Check sheet for the modelled part. Datum: model origin and axes. Units: mm. A direction names the side the tool comes from. Give positions to 0.01 mm unless a question says otherwise; leave off trailing zeros. Loops run counter-clockwise (first coordinate to the right, second up) from the corner with the lowest first, then second, coordinate; pieces in that order, holes last. Notation, with made-up numbers: M 46,-14.75 L 54,-14.75 A24 cw 54,15.25 Z; hole C 46.25,80.25 d3. An arc over 180 degrees is marked long. One line per question, with ' | ' between items. Start each with the question number.
from build123d import *

# Parameters (mm, degrees)
CUT_EXTRUDE1_START     = -4
CUT_EXTRUDE1_OUTLINE_R = 1
CUT_EXTRUDE1_DEPTH     = 4
SKETCH3_R              = 1
CUT_EXTRUDE2_DEPTH     = 3


# Read off the part's stored shape, not the designer's step: Cut-Extrude1
with BuildPart() as part:
    # Sketch1 → Revolve1 (revolve)
    with BuildSketch(Plane.XY, mode=Mode.PRIVATE) as revolve1_sk:
        Polygon((0, 22), (0, -1.8), (1, -1.8), (1, 0), (9.5, 0), (11.5, 2), (11.5, 3), (11, 3), (11, 3.5), (11.5, 3.5), (11.5, 4.5), (9.5, 4.5), (9.5, 4.8), (11.5, 4.8), (11.5, 14.5), (7.5, 18.5), (1, 18.5), (1, 22), align=None)
        Polygon((2, 17.5), (7.085786438, 17.5), (10.5, 14.085786438), (10.5, 11.635505843), (1, 11.635505843), (1, 16.5), (2, 16.5), align=None, mode=Mode.SUBTRACT)
    revolve(revolve1_sk.sketch.rotate(Axis((0, 22, 0), (0, -1, 0)), 180), axis=Axis((0, 22, 0), (0, -1, 0)))

    # Cut-Extrude1 outline → Cut-Extrude1 (cut)
    with BuildSketch(Plane(origin=(0, 18.5, 0), x_dir=(1, 0, 0), z_dir=(0, 1, 0)).offset(CUT_EXTRUDE1_START)):
        with BuildLine():
            Line((-3, 14.723214578), (-3, 9))
            ThreePointArc((-3, 9), (-2.83069097, 8.006426333), (-2.341874246, 7.124999996))
            ThreePointArc((-2.341874246, 7.124999996), (0, 7.5), (2.341874249, 7.125))
            ThreePointArc((2.341874249, 7.125), (2.830690966, 8.006426323), (3, 9))
            Line((3, 9), (3, 14.723214578))
            Line((3, 14.723214578), (-3, 14.723214578))
        make_face()
        with BuildLine():
            Line((11.25067785, 9.9596835), (6.294228634, 7.098076211))
            ThreePointArc((6.294228634, 7.098076211), (5.518423113, 6.454663457), (4.999493876, 5.590622588))
            ThreePointArc((4.999493876, 5.590622588), (6.495190528, 3.75), (7.341368127, 1.534377408))
            ThreePointArc((7.341368127, 1.534377408), (8.349114075, 1.551762875), (9.294228634, 1.901923789))
            Line((9.294228634, 1.901923789), (14.25067785, 4.763531077))
            Line((14.25067785, 4.763531077), (11.25067785, 9.9596835))
        make_face()
        with BuildLine():
            Line((14.25067785, -4.763531077), (9.294228634, -1.901923789))
            ThreePointArc((9.294228634, -1.901923789), (8.349114084, -1.551762876), (7.341368122, -1.534377408))
            ThreePointArc((7.341368122, -1.534377408), (6.495190528, -3.75), (4.999493877, -5.590622592))
            ThreePointArc((4.999493877, -5.590622592), (5.518423107, -6.45466345), (6.294228634, -7.098076211))
            Line((6.294228634, -7.098076211), (11.25067785, -9.9596835))
            Line((11.25067785, -9.9596835), (14.25067785, -4.763531077))
        make_face()
        with BuildLine():
            Line((3, -14.723214578), (3, -9))
            ThreePointArc((3, -9), (2.83069097, -8.006426333), (2.341874246, -7.124999996))
            ThreePointArc((2.341874246, -7.124999996), (0, -7.5), (-2.341874249, -7.125))
            ThreePointArc((-2.341874249, -7.125), (-2.830690966, -8.006426323), (-3, -9))
            Line((-3, -9), (-3, -14.723214578))
            Line((-3, -14.723214578), (3, -14.723214578))
        make_face()
        with BuildLine():
            Line((-11.25067785, -9.9596835), (-6.294228634, -7.098076211))
            ThreePointArc((-6.294228634, -7.098076211), (-5.518423113, -6.454663457), (-4.999493876, -5.590622588))
            ThreePointArc((-4.999493876, -5.590622588), (-6.495190528, -3.75), (-7.341368127, -1.534377408))
            ThreePointArc((-7.341368127, -1.534377408), (-8.349114075, -1.551762875), (-9.294228634, -1.901923789))
            Line((-9.294228634, -1.901923789), (-14.25067785, -4.763531077))
            Line((-14.25067785, -4.763531077), (-11.25067785, -9.9596835))
        make_face()
        with BuildLine():
            Line((-14.25067785, 4.763531077), (-9.294228634, 1.901923789))
            ThreePointArc((-9.294228634, 1.901923789), (-8.349114084, 1.551762876), (-7.341368122, 1.534377408))
            ThreePointArc((-7.341368122, 1.534377408), (-6.495190528, 3.75), (-4.999493877, 5.590622592))
            ThreePointArc((-4.999493877, 5.590622592), (-5.518423107, 6.45466345), (-6.294228634, 7.098076211))
            Line((-6.294228634, 7.098076211), (-11.25067785, 9.9596835))
            Line((-11.25067785, 9.9596835), (-14.25067785, 4.763531077))
        make_face()
        with Locations((0, 4.5)):
            Circle(CUT_EXTRUDE1_OUTLINE_R)
        with Locations((4.5, 0)):
            Circle(CUT_EXTRUDE1_OUTLINE_R)
        with Locations((0, -4.5)):
            Circle(CUT_EXTRUDE1_OUTLINE_R)
        with Locations((-4.5, 0)):
            Circle(CUT_EXTRUDE1_OUTLINE_R)
    extrude(amount=CUT_EXTRUDE1_DEPTH, mode=Mode.SUBTRACT)

    # Sketch3 → Cut-Extrude2 (cut)
    with BuildSketch(Plane.XZ):
        with Locations((0, 6)):
            Circle(SKETCH3_R)
        with Locations((0, -6)):
            Circle(SKETCH3_R)
        with Locations((8, 0)):
            Circle(SKETCH3_R)
        with Locations((-8, 0)):
            Circle(SKETCH3_R)
    extrude(amount=-CUT_EXTRUDE2_DEPTH, mode=Mode.SUBTRACT)


solid = part.part
Q1. Material ranges on probe 1 along Y at (x, z) = (1, 5.75); probe 2 along Z at (x, y) = (0, 18.2); probe 3 along Z at (x, y) = (8, 1.2), recorded low to high. Write a range as from..to.
Q2. Cross-section at C-C (x = 0). State how many separate pieces and enclosed holes the cut face has, and give its area (3 significant figures).
Q3. Cross-section at B-B (y = 7.5). Record the cut outline in (x, z).
Q4. Depth check by flat-ended pin: P1, Ø1.8, axis at x = 0, z = 4.5, coming from the +Y side; P2, Ø4, axis at x = 9, z = -3.5, coming from the +Y side; P3, Ø4, axis at x = -4.5, y = 1, coming from the +Z side. Enter the tip coordinate at first touch or a pass-through.
Q5. Access from +Z, -Z, +X, -X, +Y, -Y to the whole of each face (thin tool, end or side, straight path). Record for faces 4 (the flat face through (-7.01, 15.27, 7.51)), 5 (the flat face through (-3, 15, -10)), 6 (the cylindrical face through (-10, 12.8, -3.2)), 7 (the cylindrical face through (8.363, 16.776, 1.554)).
Q6. Cross-section at A-A (y = 0.5). Record the cut outline in (x, z), and give its area (3 significant figures).
Q7. Cross-section at D-D (y = 18). Record the cut outline in (x, z) (1 decimal).
Q8. Draft check along X on faces 1 (the cylindrical face through (-0.13, 17.99, -5.49)), 2 (the flat face through (0, 22, 0)), 3 (the cylindrical face through (-5.509, 16.776, -6.444)). Enter one of: released by +X, released by -X, zero draft, split by the parting line, or undercut.
Solved:
1) probe 1: y = 0..11.64, 17.5..18.5 | probe 2: z = -7.5..-5.5, -3.5..3.5, 5.5..7.5 | probe 3: z = -7.11..-1, 1..7.11
2) separate pieces: 3 | enclosed holes: 0 | area: 291 mm²
3) outline: C 0,0 d23
4) P1: stops at y = 11.64 | P2: stops at y = 17.4 | P3: stops at z = 11.16
5) face 4: -X, +Y | face 5: -Z, +Y | face 6: none | face 7: +Z, +Y
6) outline: C 0,0 d20; hole C -8,0 d2; hole C 0,-6 d2; hole C 0,6 d2; hole C 8,0 d2 | area: 302 mm²
7) outline: M -7.9,-1.5 A3 cw -7.3,-1.5 A7.5 ccw -5,-5.6 A3 cw -5.2,-6.1 A8 ccw -2.6,-7.6 A3 cw -2.3,-7.1 A7.5 ccw 2.3,-7.1 A3 cw 2.6,-7.6 A8 ccw 5.2,-6.1 A3 cw 5,-5.6 A7.5 ccw 7.3,-1.5 A3 cw 7.9,-1.5 A8 ccw 7.9,1.5 A3 cw 7.3,1.5 A7.5 ccw 5,5.6 A3 cw 5.2,6.1 A8 ccw 2.6,7.6 A3 cw 2.3,7.1 A7.5 ccw -2.3,7.1 A3 cw -2.6,7.6 A8 ccw -5.2,6.1 A3 cw -5,5.6 A7.5 ccw -7.3,1.5 A3 cw -7.9,1.5 A8 ccw Z; hole C -4.5,0 d2; hole C 0,-4.5 d2; hole C 0,4.5 d2; hole C 4.5,0 d2
8) face 1: undercut | face 2: zero draft | face 3: released by -X
